```python
from build123d import *

# Parameters (mm, degrees)
BOSS_EXTRUDE1_DEPTH = 50
SKETCH3_W           = 14.282150027
SKETCH3_H           = 50
BOSS_EXTRUDE2_DEPTH = 100
CUT_EXTRUDE3_START  = -200
SKETCH10_R          = 55
CUT_EXTRUDE3_DEPTH  = 200
SKETCH11_W          = 91.379110146
SKETCH11_H          = 50
BOSS_EXTRUDE4_DEPTH = 80
CUT_EXTRUDE4_START  = -200
SKETCH12_R          = 55
CUT_EXTRUDE4_DEPTH  = 200


with BuildPart() as part:
    # Sketch1 → Boss-Extrude1 (new body)
    with BuildSketch(Plane(origin=(0, 0, 0), x_dir=(1, 0, 0), z_dir=(0, 1, 0))):
        with BuildLine():
            ThreePointArc((-70, 0), (0, -70), (70, 0))
            Line((70, 0), (55, 0))
            ThreePointArc((55, 0), (0, -55), (-55, 0))
            Line((-55, 0), (-70, 0))
        make_face()
    extrude(amount=BOSS_EXTRUDE1_DEPTH)

    # Sketch3 → Boss-Extrude2 (add, symmetric)
    with BuildSketch(Plane(origin=(0, 0, 0), x_dir=(0, 0, -1), z_dir=(1, 0, 0))):
        with Locations((-7.141075014, 25)):
            Rectangle(SKETCH3_W, SKETCH3_H)
    extrude(amount=BOSS_EXTRUDE2_DEPTH, both=True)

    # Sketch10 → Cut-Extrude3 (cut)
    with BuildSketch(Plane(origin=(0, 50, 0), x_dir=(1, 0, 0), z_dir=(0, 1, 0)).offset(CUT_EXTRUDE3_START)):
        Circle(SKETCH10_R)
    extrude(amount=CUT_EXTRUDE3_DEPTH, mode=Mode.SUBTRACT)

    # Sketch11 → Boss-Extrude4 (add)
    with BuildSketch(Plane.XY):
        with Locations((0, 25)):
            Rectangle(SKETCH11_W, SKETCH11_H)
    extrude(amount=BOSS_EXTRUDE4_DEPTH)

    # Sketch12 → Cut-Extrude4 (cut)
    with BuildSketch(Plane(origin=(0, 50, 0), x_dir=(1, 0, 0), z_dir=(0, 1, 0)).offset(CUT_EXTRUDE4_START)):
        Circle(SKETCH12_R)
    extrude(amount=CUT_EXTRUDE4_DEPTH, mode=Mode.SUBTRACT)


solid = part.part
```
Geometry: final body of the model. Coordinates: model frame, mm. A direction names the side the tool comes from. Coordinates: 2 decimals unless noted, no trailing zeros. Loops run counter-clockwise (first coordinate to the right, second up) from the corner with the lowest first, then second, coordinate; pieces in that order, holes last. Notation, with made-up numbers: M 25.5,40.25 L 69.5,40.25 A13 cw 69.5,60.25 Z; hole C 74.5,82 d9. An arc over 180 degrees is marked long. Put each result on its own line as item: value.
(1) Draft query along X for faces 4 (the face through (-45.69, 25, 66)), 5 (the face through (-8, 0, 55)), 6 (the face through (-1.209, 24.65, 54.987)), 7 (the face through (60.14, 24.65, 35.82)). Return one class per face: pulls with the +X half, pulls with the -X half, needs draft (parallel to the pull), parting line crosses it, or undercut.
Answer sheet:
face 4: pulls with the -X half
face 5: needs draft
face 6: undercut
face 7: pulls with the +X half
(2) Cut plane D-D on z = 59. Return the cut outline in (x, y), then the cut area to 3 significant figures.
Answer sheet:
outline: M -45.69,0 L 45.69,0 L 45.69,50 L -45.69,50 Z
area: 4,570 mm^2
(3) Cut plane C-C on x = 0. Return the cut outline in (y, z), then the cut area to 3 significant figures.
Answer sheet:
outline: M 0,55 L 50,55 L 50,80 L 0,80 Z
area: 1,250 mm^2
(4) First-contact query: pin 1 (2 mm diameter, centred on x = 36, y = 28, fed in from -Z); pin 2 (1 mm diameter, centred on y = 20, z = 20, fed in from +X); pin 3 (2 mm diameter, centred on x = -39.5, y = 40.5, fed in from -Z). Flat tips, straight axial feed; report the tip coordinate or a pass-through.
Answer sheet:
pin 1: stops at z = 40.69
pin 2: stops at x = 67.23
pin 3: stops at z = 37.21
(5) Material intervals for probe 1 along Z at (x, y) = (89.5, 14); probe 2 along X at (y, z) = (10, 57); probe 3 along X at (y, z) = (22.5, 32), sorted ascending.
Answer sheet:
probe 1: z = 0 to 14.28
probe 2: x = -45.69 to 45.69
probe 3: x = -62.26 to -44.73, 44.73 to 62.26
(6) Cut plane A-A on z = 27. Return the cut outline in (x, y).
Answer sheet:
outline: M -64.58,0 L -47.92,0 L -47.92,50 L -64.58,50 Z; M 47.92,0 L 64.58,0 L 64.58,50 L 47.92,50 Z
(7) Access query for faces 1 (the face through (84, 25, 14.282)), 2 (the face through (-8, 50, 55)), 3 (the face through (-84, 25, 14.282)). Directions: +Z, -Z, +X, -X, +Y, -Y. A direction counts if a zero-diameter tool reaches every point of the face in a straight line with its end or side. Return the directions, or none.
Answer sheet:
face 1: +Z, +X, +Y, -Y
face 2: +Z, -Z, +X, -X, +Y
face 3: +Z, -X, +Y, -Y
(8) Cut plane B-B on y = 9. Return the cut outline in (x, z), then the cut area to 3 significant figures.
Answer sheet:
outline: M -100,0 L -55,0 A55 cw 55,0 L 100,0 L 100,14.28 L 68.53,14.28 A70 ccw 45.69,53.03 L 45.69,80 L -45.69,80 L -45.69,53.03 A70 ccw -68.53,14.28 L -100,14.28 Z
area: 5,220 mm^2
